For this review, take the finished solid that the model builds, in its own axes (mm). A direction names the side the tool comes from. Coordinates: 2 decimals unless noted, no trailing zeros. Write each loop counter-clockwise with the first axis right and the second up, starting at its lowest first coordinate (ties: lowest second). Pieces come first, ordered by that corner, then holes.
```python
from build123d import *

# Parameters (mm, degrees)
EXTRUDE_367_DEPTH      = 13.5
EXTRUDE_367_DEPTH_BACK = 13.5
SKETCH_1_W             = 34
SKETCH_1_H             = 119
SKETCH_2_W             = 20
SKETCH_2_H             = 27
EXTRUDE_574_DEPTH      = 7
CHAMFER_1_SIZE         = 10
CHAMFER_1_SIZE2        = 3
FILLET_2_R             = 10
FILLET_3_R             = 5
FILLET_4_R             = 2


with BuildPart() as part:
    # Эскиз1 → Extrude 367 (new, two sides: drawn at the far end of the back side and taken through both)
    with BuildSketch(Plane(origin=(0, 0, 0), x_dir=(1, 0, 0), z_dir=(0, 1, 0)).offset(-EXTRUDE_367_DEPTH_BACK)):
        Rectangle(SKETCH_1_W, SKETCH_1_H)
    extrude(amount=EXTRUDE_367_DEPTH + EXTRUDE_367_DEPTH_BACK)

    # Эскиз2 → Extrude 574 (add)
    with BuildSketch(Plane(origin=(17, 0, 0), x_dir=(0, 0, -1), z_dir=(1, 0, 0))):
        with Locations((62.5, 0)):
            Rectangle(SKETCH_2_W, SKETCH_2_H)
    extrude(amount=EXTRUDE_574_DEPTH)

    # Фаска1
    chamfer_1_edges = [part.edges().sort_by_distance(p)[0] for p in [
        (17, 0, -59.5),
    ]]
    chamfer_1_side = [part.faces().sort_by_distance(p)[0] for p in [
        (0, 0, -59.5),
    ]]
    chamfer(chamfer_1_edges, length=CHAMFER_1_SIZE, length2=CHAMFER_1_SIZE2, reference=chamfer_1_side[0])

    # Скругление2
    # the kernel refuses this fillet: 10 mm, written as the material it adds along each edge
    with BuildSketch(Plane(origin=(7, 13.5, -59.5), x_dir=(-1, 0, 0), z_dir=(0, -1, 0))) as fillet_2_piece_1:
        with BuildLine():
            CenterArc((FILLET_2_R * 0.146768836304, FILLET_2_R), FILLET_2_R, 253.300755766, 16.699244234)
            Line((-FILLET_2_R * 0.140579049263, FILLET_2_R * 0.0421737147788), (0, 0))
            Line((0, 0), (FILLET_2_R * 0.146768836304, 0))
        make_face()
    extrude(amount=27)
    # the kernel refuses this fillet: 10 mm, written as the material it takes off along each edge
    with BuildSketch(Plane(origin=(24, -37.348480035, -52.5), x_dir=(0, 0, -1), z_dir=(0, 1, 0))) as fillet_2_2_piece_1:
        with BuildLine():
            CenterArc((9.539392014, 10), FILLET_2_R, 197.457603124, 72.542396876)
            Line((0, 7), (0, 0))
            Line((0, 0), (9.539392014, 0))
        make_face()
    extrude(amount=74.696960071, mode=Mode.SUBTRACT)

    # Скругление3
    fillet_3_edges = [part.edges().sort_by_distance(p)[0] for p in [
        (17, 0, -52.5),
    ]]
    fillet(fillet_3_edges, radius=FILLET_3_R)

    # Скругление4
    fillet_4_edges = [part.edges().sort_by_distance(p)[0] for p in [
        (17, 0, -62.5),
    ]]
    fillet(fillet_4_edges, radius=FILLET_4_R)


solid = part.part
```
1) Clearance check with flat-ended pins moving along their axes: P1, Ø8, axis at y = -4, z = 18, coming from the +X side; P2, Ø4.5, axis at y = 6.5, z = -66, coming from the -X side. State where each tip first meets the part, or that it passes through.
2) Consider section A-A (y = -7.25). Give the boundary of the cut face in (x, z).
3) Tool access review of faces 1 (the face through (-6, 0, -59.5)), 2 (the face through (17, 0, 6)), 3 (the face through (0, 0, 59.5)): name each direction out of +Z, -Z, +X, -X, +Y, -Y from which nothing blocks a thin tool from reaching the whole face with its end or side.
4) Consider section C-C (z = 45.5). Give the boundary of the cut face in (x, y), then the cut area to 3 significant figures.
5) For L1, parallel to X at y = 12, z = -11; L2, parallel to Z at x = -4, y = 3.75; L3, parallel to Z at x = 11.5, y = 3, list the stretches that pass through material, from the lowest coordinate up.
6) Consider section B-B (x = 10.5). Give the boundary of the cut face in (y, z), then the cut area to 3 significant figures.
Results:
1. P1: stops at x = 17
1. P2: stops at x = 16.99
2. outline: (-17, -59.5) - (5.53, -59.5) arc R10 cw to (8.41, -59.92) - (15.57, -62.07) arc R2 cw to (17, -63.99) - (17, -72.5) - (24, -72.5) - (24, -62.04) arc R10 ccw to (19.33, -53.58) arc R5 cw to (17, -49.35) - (17, 59.5) - (-17, 59.5) - close
3. face 1: -Z, -X, +Y, -Y
3. face 2: +Z, +X, +Y, -Y
3. face 3: +Z, +X, -X, +Y, -Y
4. outline: (-17, -13.5) - (17, -13.5) - (17, 13.5) - (-17, 13.5) - close
4. area: 918 mm2
5. L1: x = -17 to 17
5. L2: z = -59.5 to 59.5
5. L3: z = -60.85 to 59.5
6. outline: (-13.5, -60.55) - (13.5, -60.55) - (13.5, 59.5) - (-13.5, 59.5) - close
6. area: 3,240 mm2
